```python
from build123d import *

# Parameters (mm, degrees)
F0_W          = 25.4
F0_H          = 38.1
F1_DEPTH      = 171.45
F1_DEPTH_BACK = 171.45
F3_D          = 17.4625
F5_DEPTH      = 25.4


with BuildPart() as f1:
    # F0 (on Front) → F1 (new body, two sides)
    with BuildSketch(Plane.XZ) as f1_sk:
        Rectangle(F0_W, F0_H)
    extrude(amount=F1_DEPTH)
    extrude(f1_sk.sketch, amount=-F1_DEPTH_BACK)

    # F3 (through all)
    with Locations(Plane.YZ.offset(12.7)):
        with Locations((152.908, 0)):
            Hole(F3_D / 2)

    # F4 (on face) → F5 (cut)
    with BuildSketch(Plane.YZ.offset(12.7)):
        with BuildLine():
            Line((-144.17675, -19.05), (-144.17675, 0))
            ThreePointArc((-144.17675, 0), (-152.908, 8.73125), (-161.63925, 0))
            Line((-161.63925, 0), (-161.63925, -19.05))
            Line((-161.63925, -19.05), (-144.17675, -19.05))
        make_face()
    extrude(amount=-F5_DEPTH, mode=Mode.SUBTRACT)


solid = f1.part
```
Part model, mm, in its own coordinate system. A direction names the side the tool comes from. Round coordinates to 2 decimals unless told otherwise and drop trailing zeros. Order: outer loops, then holes, each group sorted by start corner. A loop starts at its lowest first (then second) coordinate and runs counter-clockwise, first axis right, second up. Notation, with made-up numbers: M 40,63 L 86,63 A30 ccw 86,86 Z; hole C 57,-39 d2. An arc over 180 degrees is marked long. Put each result on its own line as item: value. Start each with the question number.
1. Slice it at B-B on z = 4.5. List the corners of the cut face in (x, y).
2. Drill centre lines: probe 1 along Y at (x, z) = (-5.75, -6.5); probe 2 along Y at (x, z) = (-3, -2); probe 3 along Z at (x, y) = (-4.75, -152). Where is each one in solid material? Low to high. Write a range as [from, to].
3. Slice it at A-A on x = -9. List the corners of the cut face in (y, z).
4. Two-plate mould, pull along Y, no slides. Class faces 3 (the face through (0, -167, -19.05)), 4 (the face through (0, 171.45, 0)), 5 (the face through (0.18, -152.72, 8.73)): +Y half, -Y half, draft (parallel to the pull), parting line (faces both ways), or undercut.
5. Tool access for faces 1 (the face through (0, -161.639, -9)), 2 (the face through (0, -2, 19.05)): list every direction of +Z, -Z, +X, -X, +Y, -Y with a clear straight run to the whole face (end or side of a thin tool).
Findings:
1. outline: M -12.7,-171.45 L 12.7,-171.45 L 12.7,-160.39 L -12.7,-160.39 Z; M -12.7,-145.43 L 12.7,-145.43 L 12.7,145.43 L -12.7,145.43 Z; M -12.7,160.39 L 12.7,160.39 L 12.7,171.45 L -12.7,171.45 Z
2. probe 1: [-171.45, -161.64], [-144.18, 147.08], [158.74, 171.45]
2. probe 2: [-171.45, -161.64], [-144.18, 144.41], [161.41, 171.45]
2. probe 3: [8.68, 19.05]
3. outline: M -171.45,-19.05 L -161.64,-19.05 L -161.64,0 A8.73 cw -144.18,0 L -144.18,-19.05 L 171.45,-19.05 L 171.45,19.05 L -171.45,19.05 Z; hole C 152.91,0 d17.46
4. face 3: draft
4. face 4: +Y half
4. face 5: undercut
5. face 1: -Z, +X, -X
5. face 2: +Z, +X, -X, +Y, -Y
